Could you check a few things on this model? Use its own coordinates, in mm. A direction names the side the tool comes from. Give positions to 0.01 mm unless a question says otherwise; leave off trailing zeros. Order: outer loops, then holes, each group sorted by start corner. A loop starts at its lowest first (then second) coordinate and runs counter-clockwise, first axis right, second up. Notation, with made-up numbers: M 60.5,-5 L 80.5,-5 A4 ccw 80.5,-1 Z; hole C -35,-6 d1. An arc over 180 degrees is marked long. Return JSON: item names as keys, results as strings. Group by question number.
```python
from build123d import *

# Parameters (mm, degrees)
SKETCH1_W           = 63.5
SKETCH1_H           = 21.59
BOSS_EXTRUDE1_DEPTH = 5.08
SKETCH2_W           = 19.05
SKETCH2_H           = 20.32
BOSS_EXTRUDE2_DEPTH = 1.27
SKETCH3_W           = 1.27
SKETCH3_H           = 21.59
BOSS_EXTRUDE3_DEPTH = 20.32
SKETCH4_W           = 1.336000662
SKETCH4_H           = 43.13668157
BOSS_EXTRUDE4_DEPTH = 20.32
SKETCH5_W           = 10.16
SKETCH5_H           = 20.215193183
CUT_EXTRUDE2_DEPTH  = 1.27
SKETCH6_W           = 21.656000662
SKETCH6_H           = 1.342156596
CUT_EXTRUDE3_DEPTH  = 20.32


with BuildPart() as part:
    # Sketch1 → Boss-Extrude1 (new body)
    with BuildSketch(Plane(origin=(0, 0, 0), x_dir=(1, 0, 0), z_dir=(0, 1, 0))):
        with Locations((-28.979219315, -15.643333637)):
            Rectangle(SKETCH1_W, SKETCH1_H)
    boss_extrude1 = extrude(amount=BOSS_EXTRUDE1_DEPTH)

    # Sketch2 → Boss-Extrude2 (add)
    with BuildSketch(Plane.XY.offset(26.438333637)):
        with Locations((-28.979219315, 15.24)):
            Rectangle(SKETCH2_W, SKETCH2_H)
    boss_extrude2 = extrude(amount=-BOSS_EXTRUDE2_DEPTH)

    # Sketch3 → Boss-Extrude3 (add)
    with BuildSketch(Plane(origin=(0, 5.08, 0), x_dir=(1, 0, 0), z_dir=(0, 1, 0))):
        with Locations((-39.139219315, -15.643333637)):
            Rectangle(SKETCH3_W, SKETCH3_H)
    boss_extrude3 = extrude(amount=BOSS_EXTRUDE3_DEPTH)

    # Mirror2: Boss-Extrude1, Boss-Extrude2, Boss-Extrude3 across plane
    add(boss_extrude1.mirror(Plane(origin=(-60.729219315, 5.08, 4.848333637), x_dir=(1, 0, 0), z_dir=(0, 0, 1))))
    add(boss_extrude2.mirror(Plane(origin=(-60.729219315, 5.08, 4.848333637), x_dir=(1, 0, 0), z_dir=(0, 0, 1))))
    add(boss_extrude3.mirror(Plane(origin=(-60.729219315, 5.08, 4.848333637), x_dir=(1, 0, 0), z_dir=(0, 0, 1))))

    # Sketch4 → Boss-Extrude4 (add)
    with BuildSketch(Plane(origin=(0, 5.08, 0), x_dir=(1, 0, 0), z_dir=(0, 1, 0))):
        with Locations((-18.786218984, -4.869992852)):
            Rectangle(SKETCH4_W, SKETCH4_H)
    extrude(amount=BOSS_EXTRUDE4_DEPTH)

    # Sketch5 → Cut-Extrude2 (cut)
    with BuildSketch(Plane(origin=(0, 0, -16.741666363), x_dir=(-1, 0, 0), z_dir=(0, 0, -1))):
        with Locations((29.613387645, 15.279515477)):
            Rectangle(SKETCH5_W, SKETCH5_H)
    extrude(amount=-CUT_EXTRUDE2_DEPTH, mode=Mode.SUBTRACT)

    # Sketch6 → Cut-Extrude3 (cut)
    with BuildSketch(Plane(origin=(0, 25.4, 0), x_dir=(1, 0, 0), z_dir=(0, 1, 0))):
        with Locations((-28.946218984, 16.070588065)):
            Rectangle(SKETCH6_W, SKETCH6_H)
    extrude(amount=-CUT_EXTRUDE3_DEPTH, mode=Mode.SUBTRACT)


solid = part.part
```
1. Imagine slicing it at D-D, the plane x = -45. Please give me the cut outline in (y, z), plus the area to 3 significant figures.
2. Imagine slicing it at B-B, the plane z = -13.5. Please give me the cut outline in (x, y).
3. For pin 1 (3 mm diameter, centred on y = 7.5, z = 13, fed in from -X); pin 2 (8 mm diameter, centred on y = 22, z = -3, fed in from +X); pin 3 (1.5 mm diameter, centred on x = -18.5, y = 15, fed in from -Z), each with a flat end and sliding along its axis, tell me the tip position at first contact or that it passes through.
4. Which directions (+Z, -Z, +X, -X, +Y, -Y) give clear straight access to the entire face, cutting with the end or side of a thin tool? Please do faces 5 (the flat face through (-19.454, 15, 5)), 6 (the flat face through (-39, 15, -15.4)), 7 (the flat face through (-39.774, 15, 5)), 8 (the flat face through (-18.118, 15, 6)), 9 (the flat face through (-29, 0, 5)).
5. If we mould it in two halves opening along X, with no side actions, what happens to faces 1 (the flat face through (-29, 15, 25.168)), 2 (the flat face through (-60.729, 3, 5)), 3 (the flat face through (-29, 3, -16.742)), 4 (the flat face through (-29, 5.08, 5))? For each: pulls with the +X half, pulls with the -X half, needs draft (parallel to the pull), parting line crosses it, or undercut.
6. Imagine slicing it at A-A, the plane y = 17.75. Please give me the cut outline in (x, z), plus the area to 3 significant figures.
7. I need wall thicknesses on L1, parallel to X at y = 7.25, z = 21.5; L2, parallel to Y at x = -26, z = 9; L3, parallel to Z at x = -23, y = 8.5. Which ranges of each line are inside material? Lowest first, please. Write a range as from..to.
8. Imagine slicing it at C-C, the plane x = -37.5. Please give me the cut outline in (y, z), plus the area to 3 significant figures.
Values:
{
 "1": {"outline": "M 0,-16.74 L 5.08,-16.74 L 5.08,26.44 L 0,26.44 Z", "area": "219 mm²"},
 "2": {"outline": "M -60.73,0 L 2.77,0 L 2.77,5.08 L -18.12,5.08 L -18.12,25.4 L -19.45,25.4 L -19.45,5.08 L -38.5,5.08 L -38.5,25.4 L -39.77,25.4 L -39.77,5.08 L -60.73,5.08 Z"},
 "3": {"pin 1": "stops at x = -39.77", "pin 2": "stops at x = -18.12", "pin 3": "stops at z = -15.4"},
 "4": {"face 5": "-Z, +Y", "face 6": "-Z, +X, -X, +Y", "face 7": "+Z, -Z, -X, +Y", "face 8": "+Z, -Z, +X, +Y", "face 9": "+Z, -Z, +X, -X, -Y"},
 "5": {"face 1": "undercut", "face 2": "pulls with the -X half", "face 3": "needs draft", "face 4": "undercut"},
 "6": {"outline": "M -39.77,-15.4 L -38.5,-15.4 L -38.5,25.17 L -19.45,25.17 L -19.45,-15.4 L -18.12,-15.4 L -18.12,26.44 L -39.77,26.44 Z", "area": "133 mm²"},
 "7": {"L1": "x = -39.77..-38.5, -19.45..-18.12", "L2": "y = 0..5.08", "L3": "z = 25.17..26.44"},
 "8": {"outline": "M 0,-16.74 L 5.08,-16.74 L 5.08,25.17 L 25.4,25.17 L 25.4,26.44 L 0,26.44 Z", "area": "245 mm²"}
}
